from build123d import *

# Parameters (mm, degrees)
BOSS_EXTRUDE1_DEPTH = 4
CUT_EXTRUDE1_DEPTH  = 7.75
CUT_EXTRUDE2_DEPTH  = 7.75
SKETCH4_R           = 0.205
CUT_EXTRUDE3_DEPTH  = 2.75


with BuildPart() as part:
    # Sketch1 → Boss-Extrude1 (new, symmetric)
    with BuildSketch(Plane.XY):
        with BuildLine():
            Line((7.5, 0), (6, 0))
            ThreePointArc((6, 0), (5.439903034, -2.531295119), (3.864181673, -4.59))
            Line((3.864181673, -4.59), (7, -4.59))
            Line((7, -4.59), (7, -6.09))
            Line((7, -6.09), (-7, -6.09))
            Line((-7, -6.09), (-7, -4.59))
            Line((-7, -4.59), (-3.864181673, -4.59))
            ThreePointArc((-3.864181673, -4.59), (-5.439903034, -2.531295119), (-6, 0))
            Line((-6, 0), (-7.5, 0))
            Line((-7.5, 0), (-7.5, 0.41))
            Line((-7.5, 0.41), (7.5, 0.41))
            Line((7.5, 0.41), (7.5, 0))
        make_face()
    extrude(amount=BOSS_EXTRUDE1_DEPTH, both=True)

    # Sketch2 → Cut-Extrude1 (cut)
    with BuildSketch(Plane.XY.offset(4)):
        with BuildLine():
            Line((-4.875, 0.41), (4.875, 0.41))
            ThreePointArc((4.875, 0.41), (0, -4.465), (-4.875, 0.41))
        make_face()
    extrude(amount=-CUT_EXTRUDE1_DEPTH, mode=Mode.SUBTRACT)

    # Sketch3 → Cut-Extrude2 (cut)
    with BuildSketch(Plane(origin=(0, 0, -4), x_dir=(-1, 0, 0), z_dir=(0, 0, -1))):
        with BuildLine():
            Line((-1.5, 0.41), (1.5, 0.41))
            ThreePointArc((1.5, 0.41), (0, -1.09), (-1.5, 0.41))
        make_face()
    extrude(amount=-CUT_EXTRUDE2_DEPTH, mode=Mode.SUBTRACT)

    # Sketch4 → Cut-Extrude3 (cut)
    with BuildSketch(Plane(origin=(0, 0.41, 0), x_dir=(1, 0, 0), z_dir=(0, 1, 0))):
        with Locations(Location((6.75, 3, 0), (0, 0, 180))):
            Circle(SKETCH4_R)
        with Locations(Location((6.75, 1, 0), (0, 0, 180))):
            Circle(SKETCH4_R)
        with Locations(Location((6.75, -1, 0), (0, 0, 180))):
            Circle(SKETCH4_R)
        with Locations(Location((6.75, -3, 0), (0, 0, 180))):
            Circle(SKETCH4_R)
    cut_extrude3 = extrude(amount=-CUT_EXTRUDE3_DEPTH, mode=Mode.SUBTRACT)

    # Mirror1: Cut-Extrude3 across plane
    add(cut_extrude3.mirror(Plane(origin=(0, 0, 0), x_dir=(0, 0, 1), z_dir=(1, 0, 0))), mode=Mode.SUBTRACT)


solid = part.part
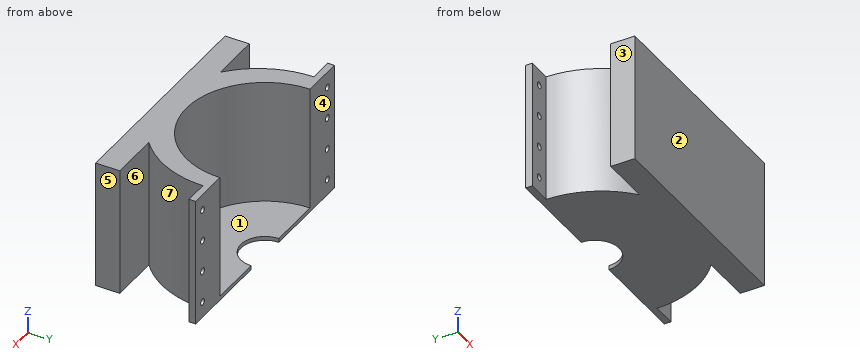
Geometry check sheet. Reference: the model listing, model coordinates, mm. Face numbers are marked on the shaded views. A direction names the side the tool comes from. Coordinates: 2 decimals unless noted, no trailing zeros. Order: outer loops, then holes, each group sorted by start corner. A loop starts at its lowest first (then second) coordinate and runs counter-clockwise, first axis right, second up. Notation, with made-up numbers: (12, 2.25) - (54, 2.25) arc R21 ccw to (54, 38.25) - close; hole circle Ø9 at (-36.75, 29). An arc over 180 degrees is marked (long way). Answer in a Markdown table with one row per item. Add a question column.
1) Material ranges on line 1 along Z through (x, y) = (-6.75, 0.3) (3 decimals); line 2 along Y through (x, z) = (-5, 2.5); line 3 along Z through (x, y) = (3.5, -1.5), recorded low to high. Write a range as [from, to].
2) Set-up check for the marked faces 1, 2 and 3: record each of +Z, -Z, +X, -X, +Y, -Y from which the full face is reachable in a straight line by a thin tool's end or side.
3) Release check for a two-part mould opening along Y. For the marked faces 4, 5, 6 and 7 record: +Y half, -Y half, draft (parallel to the pull), parting line (faces both ways), or undercut.
4) Cross-section at B-B, the plane z = -1. Record the cut outline in (x, y) (3 decimals), then the cut area to 3 significant figures.
5) Cross-section at C-C, the plane x = -4.25. Record the cut outline in (y, z).
6) Gauge pin test, flat ends, axial feed: P1, Ø2.5, axis at x = 4.5, z = 1, coming from the +Y side; P2, Ø2.5, axis at x = 0, y = -3, coming from the +Z side; P3, Ø1.2, axis at y = -5.5, z = -1.5, coming from the -X side; P4, Ø1.5, axis at y = -1, z = 1, coming from the +X side. Record the tip position at first contact, or that the pin passes through.
7) Cross-section at A-A, the plane x = -6.75. Record the cut outline in (y, z) (3 decimals), then the cut area to 3 significant figures.
8) Cross-section at D-D, the plane z = -2.5. Record the cut outline in (x, y) (3 decimals), then the cut area to 3 significant figures.
Check result:
| question | item | result |
|---|---|---|
| 1 | line 1 | z = [-4, -3.205], [-2.795, -1.205], [-0.795, 0.795], [1.205, 2.795], [3.205, 4] |
| 1 | line 2 | y = [-6.09, -4.59], [-3.32, 0.41] |
| 1 | line 3 | z = [-4, -3.75] |
| 2 | face 1 | +Z, +Y |
| 2 | face 2 | +Z, -Z, +X, -X, -Y |
| 2 | face 3 | +Z, -Z, -X, -Y |
| 3 | face 4 | +Y half |
| 3 | face 5 | draft |
| 3 | face 6 | undercut |
| 3 | face 7 | undercut |
| 4 | outline | (-7.5, 0) - (-6.955, 0) - (-6.955, 0.41) - (-7.5, 0.41) - close; (-7, -6.09) - (7, -6.09) - (7, -4.59) - (3.864, -4.59) arc R6 ccw to (6, 0) - (6.545, 0) - (6.545, 0.41) - (4.875, 0.41) arc R4.875 cw to (-4.875, 0.41) - (-6.545, 0.41) - (-6.545, 0) - (-6, 0) arc R6 ccw to (-3.864, -4.59) - (-7, -4.59) - close; (6.955, 0) - (7.5, 0) - (7.5, 0.41) - (6.955, 0.41) - close |
| 4 | area | 38.6 mm² |
| 5 | outline | (-6.09, -4) - (-4.59, -4) - (-4.59, 4) - (-6.09, 4) - close; (-4.24, -4) - (0.41, -4) - (0.41, -3.75) - (-1.98, -3.75) - (-1.98, 4) - (-4.24, 4) - close |
| 6 | P1 | stops at y = 0.41 |
| 6 | P2 | stops at z = -3.75 |
| 6 | P3 | stops at x = -7 |
| 6 | P4 | stops at x = 5.99 |
| 7 | outline | (-6.09, -4) - (-4.59, -4) - (-4.59, 4) - (-6.09, 4) - close; (0, -4) - (0.41, -4) - (0.41, -3.205) - (0, -3.205) - close; (0, -2.795) - (0.41, -2.795) - (0.41, -1.205) - (0, -1.205) - close; (0, -0.795) - (0.41, -0.795) - (0.41, 0.795) - (0, 0.795) - close; (0, 1.205) - (0.41, 1.205) - (0.41, 2.795) - (0, 2.795) - close; (0, 3.205) - (0.41, 3.205) - (0.41, 4) - (0, 4) - close |
| 7 | area | 14.6 mm² |
| 8 | outline | (-7.5, 0) - (-6, 0) arc R6 ccw to (-3.864, -4.59) - (-7, -4.59) - (-7, -6.09) - (7, -6.09) - (7, -4.59) - (3.864, -4.59) arc R6 ccw to (6, 0) - (7.5, 0) - (7.5, 0.41) - (4.875, 0.41) arc R4.875 cw to (-4.875, 0.41) - (-7.5, 0.41) - close |
| 8 | area | 38.9 mm² |
